from build123d import *

# Parameters (mm, degrees)
SKETCH1_W                = 200
SKETCH1_H                = 150
SKETCH1_W_2              = 75
SKETCH1_H_2              = 5
SKETCH1_W_3              = 15
BOSS_EXTRUDE2_DEPTH      = 10
SKETCH1_8_W              = 75
SKETCH1_8_H              = 5
SKETCH1_8_W_2            = 15
BOSS_EXTRUDE3_DEPTH      = 25
BOSS_EXTRUDE4_START      = -10
BOSS_EXTRUDE4_DEPTH      = 80
SKETCH7_R                = 5
CUT_EXTRUDE2_DEPTH       = 120
CUT_EXTRUDE2_DEPTH_BACK  = 37
CUT_EXTRUDE3_DEPTH       = 142
SKETCH9_W                = 11
SKETCH9_H                = 22
CUT_EXTRUDE4_DEPTH       = 10
SKETCH15_W               = 22
SKETCH15_H               = 11
SKETCH15_W_2             = 50
SKETCH15_H_2             = 40
CUT_EXTRUDE9_DEPTH       = 10
BOSS_EXTRUDE9_START      = -10
SKETCH18_W               = 210
SKETCH18_H               = 5
BOSS_EXTRUDE9_DEPTH      = 80
SKETCH17_W               = 16.5
SKETCH17_H               = 3
CUT_EXTRUDE11_DEPTH      = 156
CUT_EXTRUDE11_DEPTH_BACK = 6


with BuildPart() as part:
    # Sketch1 → Boss-Extrude2 (new body)
    with BuildSketch(Plane(origin=(0, 0, 0), x_dir=(1, 0, 0), z_dir=(0, 1, 0))):
        Rectangle(SKETCH1_W, SKETCH1_H)
        with Locations((46.5, -63.5)):
            Rectangle(SKETCH1_W_2, SKETCH1_H_2, mode=Mode.SUBTRACT)
        with Locations((-76.5, -63.5)):
            Rectangle(SKETCH1_W_3, SKETCH1_H_2, mode=Mode.SUBTRACT)
        with Locations((-76.5, -46.5)):
            Rectangle(SKETCH1_W_3, SKETCH1_H_2, mode=Mode.SUBTRACT)
        with Locations((46.5, -46.5)):
            Rectangle(SKETCH1_W_2, SKETCH1_H_2, mode=Mode.SUBTRACT)
        with Locations((46.5, 46.5)):
            Rectangle(SKETCH1_W_2, SKETCH1_H_2, mode=Mode.SUBTRACT)
        with Locations((46.5, 63.5)):
            Rectangle(SKETCH1_W_2, SKETCH1_H_2, mode=Mode.SUBTRACT)
        with Locations((-76.5, 63.5)):
            Rectangle(SKETCH1_W_3, SKETCH1_H_2, mode=Mode.SUBTRACT)
        with Locations((-76.5, 46.5)):
            Rectangle(SKETCH1_W_3, SKETCH1_H_2, mode=Mode.SUBTRACT)
    extrude(amount=-BOSS_EXTRUDE2_DEPTH)

    # Sketch1<8> → Boss-Extrude3 (add)
    with BuildSketch(Plane(origin=(0, 0, 0), x_dir=(1, 0, 0), z_dir=(0, 1, 0))):
        with Locations((46.5, -63.5)):
            Rectangle(SKETCH1_8_W, SKETCH1_8_H)
        with Locations((-76.5, -63.5)):
            Rectangle(SKETCH1_8_W_2, SKETCH1_8_H)
        with Locations((-76.5, -46.5)):
            Rectangle(SKETCH1_8_W_2, SKETCH1_8_H)
        with Locations((46.5, -46.5)):
            Rectangle(SKETCH1_8_W, SKETCH1_8_H)
        with Locations((46.5, 46.5)):
            Rectangle(SKETCH1_8_W, SKETCH1_8_H)
        with Locations((46.5, 63.5)):
            Rectangle(SKETCH1_8_W, SKETCH1_8_H)
        with Locations((-76.5, 63.5)):
            Rectangle(SKETCH1_8_W_2, SKETCH1_8_H)
        with Locations((-76.5, 46.5)):
            Rectangle(SKETCH1_8_W_2, SKETCH1_8_H)
    extrude(amount=-BOSS_EXTRUDE3_DEPTH)

    # Sketch5 → Boss-Extrude4 (add)
    with BuildSketch(Plane(origin=(0, 0, 0), x_dir=(-1, 0, 0), z_dir=(0, 1, 0)).offset(BOSS_EXTRUDE4_START)):
        Polygon((100, 75), (100, -75), (105, -75), (105, 70.097096622), (105, 80), (-105, 80), (-105, 70.097096622), (-105, -75), (-100, -75), (-100, 75), align=None)
    extrude(amount=BOSS_EXTRUDE4_DEPTH)

    # Sketch7 → Cut-Extrude2 (cut, two sides)
    with BuildSketch(Plane(origin=(0, 0, 44), x_dir=(-1, 0, 0), z_dir=(0, 0, -1))) as cut_extrude2_sk:
        with Locations((76.5, -17.5)):
            Circle(SKETCH7_R)
    extrude(amount=CUT_EXTRUDE2_DEPTH, mode=Mode.SUBTRACT)
    extrude(cut_extrude2_sk.sketch, amount=-CUT_EXTRUDE2_DEPTH_BACK, mode=Mode.SUBTRACT)

    # Sketch8 → Cut-Extrude3 (cut, through all)
    with BuildSketch(Plane.XY.offset(66)):
        with BuildLine():
            Line((16.5, -12.5), (76.5, -12.5))
            ThreePointArc((76.5, -12.5), (81.5, -17.5), (76.5, -22.5))
            Line((76.5, -22.5), (16.5, -22.5))
            ThreePointArc((16.5, -22.5), (11.5, -17.5), (16.5, -12.5))
        make_face()
    extrude(amount=-CUT_EXTRUDE3_DEPTH, mode=Mode.SUBTRACT)

    # Sketch9 → Cut-Extrude4 (cut)
    with BuildSketch(Plane.XY.offset(80)):
        with Locations((0, 40)):
            Rectangle(SKETCH9_W, SKETCH9_H)
    extrude(amount=-CUT_EXTRUDE4_DEPTH, mode=Mode.SUBTRACT)

    # Sketch15 → Cut-Extrude9 (cut)
    with BuildSketch(Plane.XZ.offset(10)):
        with Locations((-68.5, 2.5)):
            Rectangle(SKETCH15_W, SKETCH15_H)
        with Locations((68.5, 2.5)):
            Rectangle(SKETCH15_W, SKETCH15_H)
        Rectangle(SKETCH15_W_2, SKETCH15_H_2)
    extrude(amount=-CUT_EXTRUDE9_DEPTH, mode=Mode.SUBTRACT)

    # Sketch18 → Boss-Extrude9 (add)
    with BuildSketch(Plane(origin=(0, 0, 0), x_dir=(1, 0, 0), z_dir=(0, 1, 0)).offset(BOSS_EXTRUDE9_START)):
        with Locations((0, 77.5)):
            Rectangle(SKETCH18_W, SKETCH18_H)
    extrude(amount=BOSS_EXTRUDE9_DEPTH)

    # Sketch17 → Cut-Extrude11 (cut, two sides)
    with BuildSketch(Plane(origin=(0, 0, 75), x_dir=(-1, 0, 0), z_dir=(0, 0, -1))) as cut_extrude11_sk:
        with Locations((-85.75, 11.5)):
            Rectangle(SKETCH17_W, SKETCH17_H)
        with Locations((85.75, 11.5)):
            Rectangle(SKETCH17_W, SKETCH17_H)
    extrude(amount=CUT_EXTRUDE11_DEPTH, mode=Mode.SUBTRACT)
    extrude(cut_extrude11_sk.sketch, amount=-CUT_EXTRUDE11_DEPTH_BACK, mode=Mode.SUBTRACT)


solid = part.part
The model under review builds one solid part; all positions refer to its coordinate system, in mm. A direction names the side the tool comes from. Give positions to 0.01 mm unless a question says otherwise; leave off trailing zeros. Write each loop counter-clockwise with the first axis right and the second up, starting at its lowest first coordinate (ties: lowest second). Pieces come first, ordered by that corner, then holes.
1. Add section A-A, the plane z = 0. Write out the cut boundary in (x, y), plus the area to 3 significant figures.
2. Draft analysis for pull direction X (two halves, no side actions). For faces 6 (the flat face through (-86, 10, 77)), 7 (the flat face through (-1, 21, 80)), 8 (the flat face through (84, -17, 47)), state which applies: +X half, -X half, draft (parallel to the pull), parting line (faces both ways), or undercut.
3. Tool access review of faces 1 (the flat face through (-1, 0, 32)), 2 (the flat face through (84, -17, -46)), 3 (the flat face through (-86, 13, 77)), 4 (the flat face through (79.5, -5, 2)), 5 (the flat face through (46, -12, 61)): name each direction out of +Z, -Z, +X, -X, +Y, -Y from which nothing blocks a thin tool from reaching the whole face with its end or side.
4. For P1, Ø8, axis at x = 25.5, z = 33, coming from the -Y side; P2, Ø1.5, axis at x = 34, z = 47.5, coming from the +Y side; P3, Ø11.5, axis at x = -76.5, y = -17.5, coming from the +Z side, all flat-tipped, find the tip position at first contact; note any pin that passes through.
5. Wall thickness on L1, parallel to X at y = -17.5, z = -47.95; L2, parallel to Y at x = -76, z = -63; L3, parallel to X at y = 49.5, z = 59.5: over which ranges is each line inside the solid? List them lowest first.
6. Add section B-B, the plane y = 15.5. Write out the cut boundary in (x, z).
7. Add section D-D, the plane z = -57. Write out the cut boundary in (x, y).
8. Add section C-C, the plane y = 44.5. Write out the cut boundary in (x, z).
Worked answers:
1. outline: (-105, -10) - (-79.5, -10) - (-79.5, 0) - (-100, 0) - (-100, 70) - (-105, 70) - close; (-57.5, -10) - (-25, -10) - (-25, 0) - (-57.5, 0) - close; (25, -10) - (57.5, -10) - (57.5, 0) - (25, 0) - close; (79.5, -10) - (105, -10) - (105, 70) - (100, 70) - (100, 0) - (79.5, 0) - close
1. area: 1,860 mm2
2. face 6: undercut
2. face 7: draft
2. face 8: +X half
3. face 1: +Y
3. face 2: +Z, -Z, +X, -Y
3. face 3: +Z, -Z
3. face 4: +Y, -Y
3. face 5: +X, -X, -Y
4. P1: stops at y = -10
4. P2: stops at y = 0
4. P3: stops at z = 66
5. L1: x = -84 to -81.5, -71.5 to -69, 9 to 11.5, 81.5 to 84
5. L2: y = -25 to -22.47, -12.53 to 0
5. L3: x = -105 to -100, 100 to 105
6. outline: (-105, -80) - (105, -80) - (105, 80) - (-105, 80) - close; hole (-100, -75) - (100, -75) - (100, 75) - (-100, 75) - close
7. outline: (-105, -10) - (105, -10) - (105, 70) - (100, 70) - (100, 0) - (-100, 0) - (-100, 70) - (-105, 70) - close
8. outline: (-105, -80) - (105, -80) - (105, 80) - (5.5, 80) - (5.5, 75) - (100, 75) - (100, -75) - (-100, -75) - (-100, 75) - (-5.5, 75) - (-5.5, 80) - (-105, 80) - close
